from build123d import *

# Parameters (mm, degrees)
SKETCH2_W                                  = 146.05
SKETCH2_H                                  = 31.75
BOSS_EXTRUDE2_DEPTH                        = 9.525
SKETCH3_R                                  = 2.2479
CUT_EXTRUDE1_DEPTH                         = 11.1125
MIRROR1_AT_THE_SECOND_PLANE_COPY_1_SKETC_R = 2.2479
MIRROR1_AT_THE_SECOND_PLANE_COPY_1_DEPTH   = 11.1125


with BuildPart() as part:
    # Sketch2 → Boss-Extrude2 (new body)
    with BuildSketch(Plane.XY):
        Rectangle(SKETCH2_W, SKETCH2_H)
        with BuildLine():
            Line((-58.7375, 12.7), (-33.072916667, 12.7))
            ThreePointArc((-33.072916667, 12.7), (-32.319899299, 12.157255789), (-32.596666667, 11.27125))
            Line((-32.596666667, 11.27125), (-59.055, -8.5725))
            ThreePointArc((-59.055, -8.5725), (-59.886225791, -8.647451583), (-60.325, -7.9375))
            Line((-60.325, -7.9375), (-60.325, 11.1125))
            ThreePointArc((-60.325, 11.1125), (-59.860032015, 12.235032015), (-58.7375, 12.7))
        make_face(mode=Mode.SUBTRACT)
        with BuildLine():
            Line((-51.59375, -12.7), (-25.929166667, -12.7))
            ThreePointArc((-25.929166667, -12.7), (-24.806634652, -12.235032015), (-24.341666667, -11.1125))
            Line((-24.341666667, -11.1125), (-24.341666667, 7.9375))
            ThreePointArc((-24.341666667, 7.9375), (-24.780440875, 8.647451583), (-25.611666667, 8.5725))
            Line((-25.611666667, 8.5725), (-52.07, -11.27125))
            ThreePointArc((-52.07, -11.27125), (-52.346767368, -12.157255789), (-51.59375, -12.7))
        make_face(mode=Mode.SUBTRACT)
        with BuildLine():
            Line((17.991666667, -11.1125), (17.991666667, 7.9375))
            ThreePointArc((17.991666667, 7.9375), (17.552892458, 8.647451583), (16.721666667, 8.5725))
            Line((16.721666667, 8.5725), (-9.736666667, -11.27125))
            ThreePointArc((-9.736666667, -11.27125), (-10.013434034, -12.157255789), (-9.260416667, -12.7))
            Line((-9.260416667, -12.7), (16.404166667, -12.7))
            ThreePointArc((16.404166667, -12.7), (17.526698682, -12.235032015), (17.991666667, -11.1125))
        make_face(mode=Mode.SUBTRACT)
        with BuildLine():
            Line((-16.721666667, -8.5725), (9.736666667, 11.27125))
            ThreePointArc((9.736666667, 11.27125), (10.013434034, 12.157255789), (9.260416667, 12.7))
            Line((9.260416667, 12.7), (-16.404166667, 12.7))
            ThreePointArc((-16.404166667, 12.7), (-17.526698682, 12.235032015), (-17.991666667, 11.1125))
            Line((-17.991666667, 11.1125), (-17.991666667, -7.9375))
            ThreePointArc((-17.991666667, -7.9375), (-17.552892458, -8.647451583), (-16.721666667, -8.5725))
        make_face(mode=Mode.SUBTRACT)
        with BuildLine():
            Line((60.325, -11.1125), (60.325, 7.9375))
            ThreePointArc((60.325, 7.9375), (59.886225791, 8.647451583), (59.055, 8.5725))
            Line((59.055, 8.5725), (32.596666667, -11.27125))
            ThreePointArc((32.596666667, -11.27125), (32.319899299, -12.157255789), (33.072916667, -12.7))
            Line((33.072916667, -12.7), (58.7375, -12.7))
            ThreePointArc((58.7375, -12.7), (59.860032015, -12.235032015), (60.325, -11.1125))
        make_face(mode=Mode.SUBTRACT)
        with BuildLine():
            Line((25.611666667, -8.5725), (52.07, 11.27125))
            ThreePointArc((52.07, 11.27125), (52.346767368, 12.157255789), (51.59375, 12.7))
            Line((51.59375, 12.7), (25.929166667, 12.7))
            ThreePointArc((25.929166667, 12.7), (24.806634652, 12.235032015), (24.341666667, 11.1125))
            Line((24.341666667, 11.1125), (24.341666667, -7.9375))
            ThreePointArc((24.341666667, -7.9375), (24.780440875, -8.647451583), (25.611666667, -8.5725))
        make_face(mode=Mode.SUBTRACT)
        with BuildLine():
            Line((-69.5325, 12.7), (-66.9925, 12.7))
            ThreePointArc((-66.9925, 12.7), (-66.318980791, 12.421019209), (-66.04, 11.7475))
            Line((-66.04, 11.7475), (-66.04, 4.1275))
            ThreePointArc((-66.04, 4.1275), (-66.318980791, 3.453980791), (-66.9925, 3.175))
            Line((-66.9925, 3.175), (-69.5325, 3.175))
            ThreePointArc((-69.5325, 3.175), (-70.206019209, 3.453980791), (-70.485, 4.1275))
            Line((-70.485, 4.1275), (-70.485, 11.7475))
            ThreePointArc((-70.485, 11.7475), (-70.206019209, 12.421019209), (-69.5325, 12.7))
        make_face(mode=Mode.SUBTRACT)
        with BuildLine():
            Line((-66.04, -11.7475), (-66.04, -4.1275))
            ThreePointArc((-66.04, -4.1275), (-66.318980791, -3.453980791), (-66.9925, -3.175))
            Line((-66.9925, -3.175), (-69.5325, -3.175))
            ThreePointArc((-69.5325, -3.175), (-70.206019209, -3.453980791), (-70.485, -4.1275))
            Line((-70.485, -4.1275), (-70.485, -11.7475))
            ThreePointArc((-70.485, -11.7475), (-70.206019209, -12.421019209), (-69.5325, -12.7))
            Line((-69.5325, -12.7), (-66.9925, -12.7))
            ThreePointArc((-66.9925, -12.7), (-66.318980791, -12.421019209), (-66.04, -11.7475))
        make_face(mode=Mode.SUBTRACT)
        with BuildLine():
            Line((69.5325, -12.7), (66.9925, -12.7))
            ThreePointArc((66.9925, -12.7), (66.318980791, -12.421019209), (66.04, -11.7475))
            Line((66.04, -11.7475), (66.04, -4.1275))
            ThreePointArc((66.04, -4.1275), (66.318980791, -3.453980791), (66.9925, -3.175))
            Line((66.9925, -3.175), (69.5325, -3.175))
            ThreePointArc((69.5325, -3.175), (70.206019209, -3.453980791), (70.485, -4.1275))
            Line((70.485, -4.1275), (70.485, -11.7475))
            ThreePointArc((70.485, -11.7475), (70.206019209, -12.421019209), (69.5325, -12.7))
        make_face(mode=Mode.SUBTRACT)
        with BuildLine():
            Line((66.04, 11.7475), (66.04, 4.1275))
            ThreePointArc((66.04, 4.1275), (66.318980791, 3.453980791), (66.9925, 3.175))
            Line((66.9925, 3.175), (69.5325, 3.175))
            ThreePointArc((69.5325, 3.175), (70.206019209, 3.453980791), (70.485, 4.1275))
            Line((70.485, 4.1275), (70.485, 11.7475))
            ThreePointArc((70.485, 11.7475), (70.206019209, 12.421019209), (69.5325, 12.7))
            Line((69.5325, 12.7), (66.9925, 12.7))
            ThreePointArc((66.9925, 12.7), (66.318980791, 12.421019209), (66.04, 11.7475))
        make_face(mode=Mode.SUBTRACT)
    extrude(amount=BOSS_EXTRUDE2_DEPTH)

    # Sketch3 → Cut-Extrude1 (cut)
    with BuildSketch(Plane.ZY.offset(73.025)):
        with Locations((4.7625, 7.9375)):
            Circle(SKETCH3_R)
    cut_extrude1 = extrude(amount=-CUT_EXTRUDE1_DEPTH, mode=Mode.SUBTRACT)

    # Mirror1: Cut-Extrude1 across plane
    add(cut_extrude1.mirror(Plane(origin=(0, 0, 0), x_dir=(0, 0, 1), z_dir=(1, 0, 0))), mode=Mode.SUBTRACT)

    # Mirror1 at the second plane: Cut-Extrude1 across plane
    add(cut_extrude1.mirror(Plane.ZX), mode=Mode.SUBTRACT)

    # Mirror1 at the second plane copy 1 sketc → Mirror1 at the second plane copy 1 (cut)
    with BuildSketch(Plane(origin=(73.025, 0, 0), x_dir=(0, 0, 1), z_dir=(1, 0, 0))):
        with Locations((4.7625, 7.9375)):
            Circle(MIRROR1_AT_THE_SECOND_PLANE_COPY_1_SKETC_R)
    extrude(amount=-MIRROR1_AT_THE_SECOND_PLANE_COPY_1_DEPTH, mode=Mode.SUBTRACT)


solid = part.part
Can you work these out from the model? Positions are in its coordinate system, mm. A direction names the side the tool comes from. Give positions to 0.01 mm unless a question says otherwise; leave off trailing zeros. Write each loop counter-clockwise with the first axis right and the second up, starting at its lowest first coordinate (ties: lowest second). Pieces come first, ordered by that corner, then holes. Notation, with made-up numbers: (-13, -36.5) -> (17, -36.5) arc R26 cw to (17, -12.5) -> close; hole circle Ø2 at (-29, 87.25). An arc over 180 degrees is marked (long way). Answer as a JSON object with one key per item and string values. Group by question number.
Item 1: Suppose I cut it at C-C (z = 1.25). State how many separate pieces and enclosed holes the cut face has, plus the area to 3 significant figures.
Item 2: For faces 4 (the face through (-73.025, 0, 5)), 5 (the face through (-61.913, 8, 5)), 6 (the face through (71.773, -10.166, 4.47)), 7 (the face through (-60.325, 1, 5)), which set-ups out of +Z, -Z, +X, -X, +Y, -Y let a thin tool reach every point of the face, with its end or its side?
Item 3: Suppose I cut it at A-A (y = -1.5). Please give me the cut outline in (x, z) (3 decimals).
Item 4: Suppose I cut it at B-B (x = -47.5). Please give me the cut outline in (y, z) (3 decimals).
Item 5: I'm going to push flat-ended pins straight in: P1, Ø3.5, axis at y = 7.5, z = 4, coming from the -X side (3 decimals); P2, Ø3.5, axis at y = 7.94, z = 4.76, coming from the +X side; P3, Ø2, axis at x = -38.5, y = 8.5, coming from the +Z side. Where does each tip first touch, or does it pass through?
Item 6: Please list where these lines run through material, in increasing order: line 1 (Y direction, x = 47, z = 8) (3 decimals); line 2 (Y direction, x = -45, z = 7.5) (3 decimals); line 3 (X direction, y = -10.5, z = 6.25) (3 decimals). Write a range as [from, to].
Item 7: We'd pull the mould along Z, two halves only. Please class faces 1 (the face through (-66.04, -11, 5)), 2 (the face through (-1, 0, 0)), 3 (the face through (-71.773, 10.166, 4.47)): +Z half, -Z half, draft (parallel to the pull), parting line (faces both ways), or undercut.
Findings:
{
 "1": {"separate pieces": "1", "enclosed holes": "10", "area": "2,510 mm²"},
 "2": {"face 4": "+Z, -Z, -X, +Y, -Y", "face 5": "-X", "face 6": "+X", "face 7": "+Z, -Z"},
 "3": {"outline": "(-73.025, 0) -> (-60.325, 0) -> (-60.325, 9.525) -> (-73.025, 9.525) -> close; (-49.625, 0) -> (-39.042, 0) -> (-39.042, 9.525) -> (-49.625, 9.525) -> close; (-24.342, 0) -> (-17.992, 0) -> (-17.992, 9.525) -> (-24.342, 9.525) -> close; (-7.292, 0) -> (3.292, 0) -> (3.292, 9.525) -> (-7.292, 9.525) -> close; (17.992, 0) -> (24.342, 0) -> (24.342, 9.525) -> (17.992, 9.525) -> close; (35.042, 0) -> (45.625, 0) -> (45.625, 9.525) -> (35.042, 9.525) -> close; (60.325, 0) -> (73.025, 0) -> (73.025, 9.525) -> (60.325, 9.525) -> close"},
 "4": {"outline": "(-15.875, 0) -> (-12.7, 0) -> (-12.7, 9.525) -> (-15.875, 9.525) -> close; (-7.844, 0) -> (0.094, 0) -> (0.094, 9.525) -> (-7.844, 9.525) -> close; (12.7, 0) -> (15.875, 0) -> (15.875, 9.525) -> (12.7, 9.525) -> close"},
 "5": {"P1": "stops at x = -73.025", "P2": "stops at x = 61.91", "P3": "passes through"},
 "6": {"line 1": "y = [-15.875, -12.7], [-0.469, 7.469], [12.7, 15.875]", "line 2": "y = [-15.875, -12.7], [-5.969, 1.969], [12.7, 15.875]", "line 3": "x = [-73.025, -70.485], [-66.04, -51.042], [-24.342, -8.708], [17.992, 33.625], [60.325, 66.04], [70.485, 73.025]"},
 "7": {"face 1": "draft", "face 2": "-Z half", "face 3": "undercut"}
}
